```python
from build123d import *

# Parameters (mm, degrees)
BOSS_EXTRUDE1_DEPTH      = 8
BOSS_EXTRUDE1_DEPTH_BACK = 8
SKETCH2_R                = 5.5
CUT_EXTRUDE1_DEPTH       = 8
CUT_EXTRUDE2_DEPTH       = 16
SKETCH4_R                = 6.5
CUT_EXTRUDE3_DEPTH       = 5
SKETCH5_W                = 23.5
SKETCH5_H                = 12.6
CUT_EXTRUDE4_DEPTH       = 33
SKETCH6_R                = 0.9
CUT_EXTRUDE5_DEPTH       = 17
SKETCH7_W                = 6
SKETCH7_H                = 7
CUT_EXTRUDE6_DEPTH       = 7
SKETCH8_W                = 5
SKETCH8_H                = 7
CUT_EXTRUDE7_DEPTH       = 10
SKETCH9_R                = 0.9
CUT_EXTRUDE8_DEPTH       = 7
SKETCH10_W               = 37.5
SKETCH10_H               = 16
CUT_EXTRUDE9_DEPTH       = 10


with BuildPart() as part:
    # Sketch1 → Boss-Extrude1 (new body, two sides)
    with BuildSketch(Plane(origin=(0, 0, 0), x_dir=(1, 0, 0), z_dir=(0, 1, 0))) as boss_extrude1_sk:
        Polygon((64, -16.835969506), (47.993540801, -16.835969506), (47.993540801, 8.164030494), (55.763890835, 8.164030494), (55.763890835, 6.5), (64, 6.5), (64, 10), (-63.5, 10), (-63.5, -10), (-51.5, -22), (64, -22), align=None)
    extrude(amount=BOSS_EXTRUDE1_DEPTH)
    extrude(boss_extrude1_sk.sketch, amount=-BOSS_EXTRUDE1_DEPTH_BACK)

    # Sketch2 → Cut-Extrude1 (cut)
    with BuildSketch(Plane.ZY.offset(63.5)):
        Circle(SKETCH2_R)
    extrude(amount=-CUT_EXTRUDE1_DEPTH, mode=Mode.SUBTRACT)

    # Sketch3 → Cut-Extrude2 (cut)
    with BuildSketch(Plane(origin=(0, 8, 0), x_dir=(1, 0, 0), z_dir=(0, 1, 0))):
        Polygon((-57.5, 6), (-22.5, 6), (-22.5, -18), (-49.843145751, -18), (-57.5, -10.343145751), align=None)
    extrude(amount=-CUT_EXTRUDE2_DEPTH, mode=Mode.SUBTRACT)

    # Sketch4 → Cut-Extrude3 (cut)
    with BuildSketch(Plane(origin=(-57.5, 0, 0), x_dir=(0, 0, -1), z_dir=(1, 0, 0))):
        Circle(SKETCH4_R)
    extrude(amount=-CUT_EXTRUDE3_DEPTH, mode=Mode.SUBTRACT)

    # Sketch5 → Cut-Extrude4 (cut, through all)
    with BuildSketch(Plane(origin=(0, 0, -10), x_dir=(-1, 0, 0), z_dir=(0, 0, -1))):
        with Locations((-5.25, 0)):
            Rectangle(SKETCH5_W, SKETCH5_H)
    extrude(amount=-CUT_EXTRUDE4_DEPTH, mode=Mode.SUBTRACT)

    # Sketch6 → Cut-Extrude5 (cut)
    with BuildSketch(Plane(origin=(0, 0, -10), x_dir=(-1, 0, 0), z_dir=(0, 0, -1))):
        with Locations((8.3, 0)):
            Circle(SKETCH6_R)
        with Locations((-19, 0)):
            Circle(SKETCH6_R)
    extrude(amount=-CUT_EXTRUDE5_DEPTH, mode=Mode.SUBTRACT)

    # Sketch7 → Cut-Extrude6 (cut)
    with BuildSketch(Plane(origin=(0, 0, -10), x_dir=(-1, 0, 0), z_dir=(0, 0, -1))):
        with Locations((-50.993540801, 0)):
            Rectangle(SKETCH7_W, SKETCH7_H)
    extrude(amount=-CUT_EXTRUDE6_DEPTH, mode=Mode.SUBTRACT)

    # Sketch8 → Cut-Extrude7 (cut)
    with BuildSketch(Plane.XY.offset(22)):
        with Locations((-9, 0)):
            Rectangle(SKETCH8_W, SKETCH8_H)
    extrude(amount=-CUT_EXTRUDE7_DEPTH, mode=Mode.SUBTRACT)

    # Sketch9 → Cut-Extrude8 (cut)
    with BuildSketch(Plane(origin=(64, 0, 0), x_dir=(0, 0, -1), z_dir=(1, 0, 0))):
        with Locations((-18.998394534, 0.246992196)):
            Circle(SKETCH9_R)
        with Locations((8.299298665, -0.107896591)):
            Circle(SKETCH9_R)
    extrude(amount=-CUT_EXTRUDE8_DEPTH, mode=Mode.SUBTRACT)

    # Sketch10 → Cut-Extrude9 (cut)
    with BuildSketch(Plane(origin=(0, 0, -10), x_dir=(-1, 0, 0), z_dir=(0, 0, -1))):
        with Locations((-5.25, 0)):
            Rectangle(SKETCH10_W, SKETCH10_H)
    extrude(amount=-CUT_EXTRUDE9_DEPTH, mode=Mode.SUBTRACT)


solid = part.part
```
Here's how the part is built. I have some questions about the finished solid (model axes, mm). A direction names the side the tool comes from. Give positions to 0.01 mm unless a question says otherwise; leave off trailing zeros. Loops run counter-clockwise (first coordinate to the right, second up) from the corner with the lowest first, then second, coordinate; pieces in that order, holes last. Notation, with made-up numbers: M 11,37.5 L 31,37.5 A32 cw 31,63.5 Z; hole C 66,77 d3. An arc over 180 degrees is marked long. Put each result on its own line as item: value. Start each with the question number.
(1) I need wall thicknesses on line 1 along X through (y, z) = (-4.75, 9); line 2 along X through (y, z) = (1, 6); line 3 along Y through (x, z) = (-9, 13.5). Which ranges of each line are inside material? Lowest first, please. Write a range as [from, to].
(2) I want a section at B-B on z = -2. Please give me the cut outline in (x, y).
(3) I want a section at A-A on x = -48. Please give me the cut outline in (y, z).
(4) For faces 1 (the flat face through (-53.618, 0.112, 14.225)), 2 (the flat face through (24, 0, -5)), 3 (the cylindrical face through (-59.965, -3.955, 5.158)), 4 (the cylindrical face through (-63.01, -5.37, -1.19)), 5 (the flat face through (17, 0, 11)), which set-ups out of +Z, -Z, +X, -X, +Y, -Y let a thin tool reach every point of the face, with its end or its side?
(5) If we mould it in two halves opening along X, with no side actions, what happens to faces 6 (the flat face through (-9, 0, 12)), 7 (the flat face through (-38, 0, -10)), 8 (the flat face through (64, 0, 21)), 9 (the flat face through (5, 6.3, 11))? For each: +X half, -X half, draft (parallel to the pull), parting line (faces both ways), or undercut.
(6) I want a section at C-C on x = 5. Please give me the cut outline in (y, z).
(7) Will these pins go through, and if not, where does the flat tip stop? pin 1 Ø2 at (y, z) = (1.5, 13) entering from -X; pin 2 Ø0.5 at (y, z) = (0, 18.5) entering from +X; pin 3 Ø4 at (y, z) = (-2.5, 2) entering from +X.
Answer block:
1. line 1: [-63.5, -57.5], [-22.5, -6.5], [17, 47.99]
1. line 2: [-63.5, -62.5], [-22.5, -6.5], [17, 47.99]
1. line 3: [-8, -3.5], [3.5, 8]
2. outline: M -63.5,-8 L -57.5,-8 L -57.5,-6.18 L -62.5,-6.18 L -62.5,-5.12 L -63.5,-5.12 Z; M -63.5,5.12 L -62.5,5.12 L -62.5,6.18 L -57.5,6.18 L -57.5,8 L -63.5,8 Z; M -22.5,-8 L -13.5,-8 L -13.5,8 L -22.5,8 Z; M 24,-8 L 47.99,-8 L 47.99,8 L 24,8 Z
3. outline: M -8,-10 L 8,-10 L 8,-6 L -8,-6 Z; M -8,18 L 8,18 L 8,22 L -8,22 Z
4. face 1: +Y, -Y
4. face 2: -Z, +Y, -Y
4. face 3: none
4. face 4: -X
4. face 5: +Z, -Z
5. face 6: undercut
5. face 7: draft
5. face 8: +X half
5. face 9: undercut
6. outline: M -8,0 L -6.3,0 L -6.3,22 L -8,22 Z; M 6.3,0 L 8,0 L 8,22 L 6.3,22 Z
7. pin 1: x = -61.5
7. pin 2: x = 57
7. pin 3: x = 47.99
